CAD build for the part. Positions are in the model's coordinates, mm. Face numbers are marked on the shaded views. Coordinates: 2 decimals unless noted, no trailing zeros. Write each loop counter-clockwise with the first axis right and the second up, starting at its lowest first coordinate (ties: lowest second). Pieces come first, ordered by that corner, then holes. Notation, with made-up numbers: (67.25, -30) - (103.25, -30) arc R20 ccw to (103.25, -19) - close; hole circle Ø3 at (-28, 85). An arc over 180 degrees is marked (long way). Answer in a Markdown table with one row per item. Add a question column.
Q1. Two-plate mould, pull along X, no slides. Class the marked faces 1, 2, 3 and 4: +X half, -X half, draft (parallel to the pull), parting line (faces both ways), or undercut.
Q2. Band-saw the part on C-C (y = 6.25). List the corners of the cut face in (x, z).
Q3. Drill centre lines: line 1 along X through (y, z) = (2.5, 0); line 2 along X through (y, z) = (1.25, 2.75); line 3 along Y through (x, z) = (-14, -3.7). Where is each one in solid material? Low to high. Write a range as from..to.
Q4. Band-saw the part on A-A (z = 0). List the corners of the cut face in (x, y).
Q5. Band-saw the part on B-B (x = 0). List the corners of the cut face in (y, z).
Q6. Band-saw the part on D-D (y = 4). List the corners of the cut face in (x, z).
Q7. Pin check, flat tips, straight feed: pin 1 (1.5 mm diameter, centred on x = 0, y = 4, fed in from -Z); pin 2 (4 mm diameter, centred on y = 2, z = 3, fed in from -X). Stop position of each tip, or through.
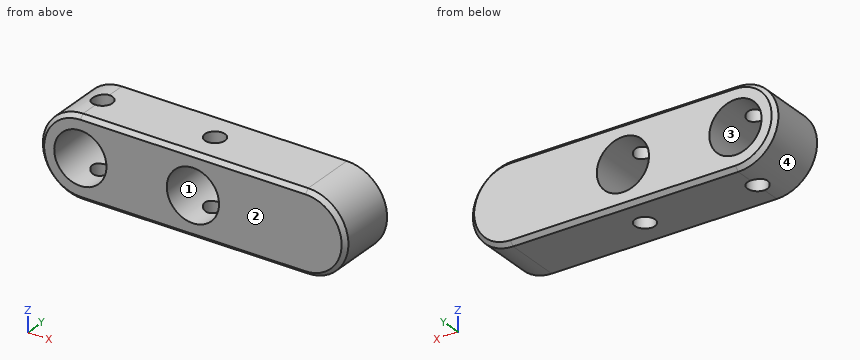
Autodesk Inventor part; units mm, degrees
ref_plane "YZ Plane" through (0, 0, 0) normal (1, 0, 0) x (0, 1, 0)
ref_plane "XZ Plane" through (0, 0, 0) normal (0, 1, 0) x (-1, 0, 0)
ref_plane "XY Plane" through (0, 0, 0) normal (0, 0, 1) x (1, 0, 0)
sketch "Skizze1" plane through (0, 0, 0) normal (0, 1, 0) x (-1, 0, 0)
  line L0 (14, 5) -> (-14, 5)
  arc A0 (-14, 5) -> (-14, -5) centre (-14, 0) ccw
  line L1 (-14, -5) -> (14, -5)
  arc A1 (14, -5) -> (14, 5) centre (14, 0) ccw
  line L2 (19, 0) -> (-19, 0) construction
  point P0 (0, 0)
  point P1 (0, 0)
  dimension "d0" = 10
  dimension "d1" = 38
extrude "Extrusion1" add sketch "Skizze1" along normal blind 8
sketch "Skizze3" plane through (0, 8, 0) normal (0, 1, 0) x (1, 0, 0)
  arc A0 (14, -5) -> (14, 5) centre (14, 0) ccw
  point P0 (0, 0)
  point P1 (0, 0)
hole "Bohrung2" at (0, 8, 0) direction (0, -1, 0) diameter 6.5 depth 8
chamfer "Fasen1" distance 0.5 angle 45 8 edges at (0, 8, -5) (-19, 8, 0) (0, 8, 5) (19, 8, 0) (0, 0, -5) (-19, 0, 0) (0, 0, 5) (19, 0, 0)
sketch "Skizze2" plane through (0, 8, 0) normal (0, 1, 0) x (1, 0, 0)
  arc A0 (-14, 5) -> (-14, -5) centre (-14, 0) ccw
  point P0 (0, 0)
  point P1 (-14, 0)
hole "Bohrung1" at (-14, 8, 0) direction (0, -1, 0) diameter 6.5 depth 8
sketch "Skizze4" plane through (14, 0, -5) normal (0, 0, -1) x (-1, 0, 0)
  line L0 (0, 8) -> (28, 8)
  line L1 (0, 0) -> (28, 0)
  line L2 (33, 0) -> (33, 8)
  line L3 (24.75, 8) -> (31.25, 8)
  line L4 (28, 0) -> (28, 8)
  point P0 (14, 0)
  point P1 (28, 4)
  point P2 (14, 4)
  point P3 (14, 0)
  point P4 (28, 4)
  dimension "d25" = 4
hole "Bohrung3" at (-14, 4, -5) at (0, 4, -5) direction (0, 0, 1) diameter 2.5 depth 10
properties part number "BMS_support" material "Gummi, Silikon"
Checked values:
| question | item | result |
|---|---|---|
| 1 | face 1 | undercut |
| 1 | face 2 | draft |
| 1 | face 3 | undercut |
| 1 | face 4 | -X half |
| 2 | outline | (-14, -5) - (14, -5) arc R5 ccw to (14, 5) - (-14, 5) arc R5 ccw to start; hole circle Ø6.5 at (-14, 0); hole circle Ø6.5 at (0, 0) |
| 3 | line 1 | x = -19..-17.25, -10.75..-3.25, 3.25..19 |
| 3 | line 2 | x = -18.18..-15.73, -12.27..-1.73, 1.73..18.18 |
| 3 | line 3 | y = 0..2.75, 5.25..8 |
| 4 | outline | (-19, 0.5) - (-18.5, 0) - (-17.25, 0) - (-17.25, 8) - (-18.5, 8) - (-19, 7.5) - close; (-10.75, 0) - (-3.25, 0) - (-3.25, 8) - (-10.75, 8) - close; (3.25, 0) - (18.5, 0) - (19, 0.5) - (19, 7.5) - (18.5, 8) - (3.25, 8) - close |
| 5 | outline | (0, -4.5) - (0.5, -5) - (2.75, -5) - (2.75, -3.25) - (0, -3.25) - close; (0, 3.25) - (2.75, 3.25) - (2.75, 5) - (0.5, 5) - (0, 4.5) - close; (5.25, -5) - (7.5, -5) - (8, -4.5) - (8, -3.25) - (5.25, -3.25) - close; (5.25, 3.25) - (8, 3.25) - (8, 4.5) - (7.5, 5) - (5.25, 5) - close |
| 6 | outline | (-15.25, -4.84) - (-15.25, -3) arc R3.25 cw to (-15.25, 3) - (-15.25, 4.84) arc R5 ccw to start; (-12.75, -5) - (-1.25, -5) - (-1.25, -3) arc R3.25 cw to (-1.25, 3) - (-1.25, 5) - (-12.75, 5) - (-12.75, 3) arc R3.25 cw to (-12.75, -3) - close; (1.25, -5) - (14, -5) arc R5 ccw to (14, 5) - (1.25, 5) - (1.25, 3) arc R3.25 cw to (1.25, -3) - close |
| 7 | pin 1 | passes through |
| 7 | pin 2 | stops at x = -18.9 |
